Check sheet for the modelled part. Datum: model origin and axes. Units: mm. A direction names the side the tool comes from. Round coordinates to 2 decimals unless told otherwise and drop trailing zeros. Write each loop counter-clockwise with the first axis right and the second up, starting at its lowest first coordinate (ties: lowest second). Pieces come first, ordered by that corner, then holes. Notation, with made-up numbers: M 53.25,23.25 L 75.25,23.25 A16 ccw 75.25,49.25 Z; hole C 67.5,50 d6. An arc over 180 degrees is marked long. Put each result on its own line as item: value.
```python
from build123d import *

# Parameters (mm, degrees)
F1_DEPTH = 51.181
F3_DEPTH = 15.24
F4_DEPTH = 3.81
F6_START = 2.54
F6_DEPTH = 8.89
F8_START = 2.54
F8_DEPTH = 20.574


with BuildPart() as f1:
    # F0 (on Right) → F1 (new body, symmetric)
    with BuildSketch(Plane.YZ):
        Polygon((8.636, 1.27), (-8.636, 1.27), (-8.636, -1.27), (-4.953, -1.27), (-4.953, -3.81), (4.953, -3.81), (4.953, -1.27), (8.636, -1.27), align=None)
    extrude(amount=F1_DEPTH, both=True)

    # F2 (on Top) → F3 (join)
    with BuildSketch(Plane.XY):
        with BuildLine():
            Line((-65.4284994702, -22.3050312109), (-33.107586205, 0))
            Line((-33.107586205, 0), (-48.0534703304, 21.6572045976))
            ThreePointArc((-48.0534703304, 21.6572045976), (-49.6859023505, 22.7128681239), (-51.5866729398, 22.3050312109))
            Line((-51.5866729398, 22.3050312109), (-81.8170715936, 1.442687998))
            ThreePointArc((-81.8170715936, 1.442687998), (-82.87273512, -0.189744022), (-82.464898207, -2.0905146114))
            Line((-82.464898207, -2.0905146114), (-68.9617020796, -21.6572045976))
            ThreePointArc((-68.9617020796, -21.6572045976), (-67.3292700595, -22.7128681239), (-65.4284994702, -22.3050312109))
        make_face()
    extrude(amount=F3_DEPTH)

    # F2 (on Top) → F4 (join)
    with BuildSketch(Plane.XY):
        with BuildLine():
            Line((-65.4284994702, -22.3050312109), (-33.107586205, 0))
            Line((-33.107586205, 0), (-48.0534703304, 21.6572045976))
            ThreePointArc((-48.0534703304, 21.6572045976), (-49.6859023505, 22.7128681239), (-51.5866729398, 22.3050312109))
            Line((-51.5866729398, 22.3050312109), (-81.8170715936, 1.442687998))
            ThreePointArc((-81.8170715936, 1.442687998), (-82.87273512, -0.189744022), (-82.464898207, -2.0905146114))
            Line((-82.464898207, -2.0905146114), (-68.9617020796, -21.6572045976))
            ThreePointArc((-68.9617020796, -21.6572045976), (-67.3292700595, -22.7128681239), (-65.4284994702, -22.3050312109))
        make_face()
    extrude(amount=-F4_DEPTH)

    # F5 (on face) → F6 (cut)
    with BuildSketch(Plane.XY.offset(1.27).offset(F6_START)):
        Polygon((-40.4348767453, 27.082724402), (-80.5502137997, -0.6013276448), (-61.860116521, -27.6840520468), (-21.7447794666, 0), align=None)
    extrude(amount=F6_DEPTH, mode=Mode.SUBTRACT)

    # F7 (on face) → F8 (cut)
    with BuildSketch(Plane.XY.offset(1.27).offset(F8_START)):
        Polygon((-40.4291285362, 20.671173085), (-72.4270038917, -1.4109259767), (-57.7466082971, -22.6834267065), (-25.7487329416, -0.6013276448), align=None)
    extrude(amount=F8_DEPTH, mode=Mode.SUBTRACT)


solid = f1.part
```
1. Release check for a two-part mould opening along Y. For faces 5 (the flat face through (51.181, 0, -1)), 6 (the flat face through (-58.59, 8.14, 13.95)), 7 (the flat face through (-67, 3, 12.7)), 8 (the cylindrical face through (-49.66, 22.71, 5.85)) record: +Y half, -Y half, draft (parallel to the pull), parting line (faces both ways), or undercut.
Computed values:
face 5: draft
face 6: undercut
face 7: undercut
face 8: +Y half
2. Access from +Z, -Z, +X, -X, +Y, -Y to the whole of each face (thin tool, end or side, straight path). Record for faces 1 (the flat face through (3, -8.636, 0)), 2 (the flat face through (-66.5, -10, 14)), 3 (the flat face through (3, -7, -1.27)), 4 (the flat face through (8, 4.953, -3)).
Computed values:
face 1: +Z, -Z, +X, -Y
face 2: +Z, +X
face 3: -Z, +X, -Y
face 4: -Z, +X, +Y
3. Cross-section at C-C (y = 11). Enter the section's corners in (x, z), then the cut area to 3 significant figures.
Computed values:
outline: M -67.97,-3.81 L -40.7,-3.81 L -40.7,3.81 L -63.74,3.81 L -63.74,12.7 L -54.44,12.7 L -54.44,15.24 L -67.97,15.24 Z
area: 280 mm2
4. Scan lines: probe 1 along Z at (x, y) = (-57, 13.5); probe 2 along Z at (x, y) = (-47, 13); probe 3 along Y at (x, z) = (-65.5, 13.5). Record each from-to range of solid material in increasing order.
Computed values:
probe 1: z = -3.81 to 3.81, 12.7 to 15.24
probe 2: z = -3.81 to 3.81
probe 3: y = -22.35 to -11.45, 3.37 to 12.7
5. Cross-section at A-A (x = 22). Enter the section's corners in (y, z).
Computed values:
outline: M -8.64,-1.27 L -4.95,-1.27 L -4.95,-3.81 L 4.95,-3.81 L 4.95,-1.27 L 8.64,-1.27 L 8.64,1.27 L -8.64,1.27 Z
6. Depth check by flat-ended pin: pin 1 Ø1.8 at (x, y) = (8.5, 7.5) entering from -Z; pin 2 Ø1.3 at (x, z) = (16, 0.5) entering from +Y; pin 3 Ø1 at (x, y) = (-11, -2) entering from +Z. Enter the tip coordinate at first touch or a pass-through.
Computed values:
pin 1: stops at z = -1.27
pin 2: stops at y = 8.64
pin 3: stops at z = 1.27
7. Cross-section at B-B (z = 10.5). Enter the section's corners in (x, y).
Computed values:
outline: M -82.46,-2.09 L -68.96,-21.66 A2.54 ccw -65.53,-22.37 L -80.55,-0.6 L -48.14,21.77 A2.54 ccw -51.59,22.31 L -81.82,1.44 A2.54 ccw Z
